Answer from the drawing. Dimensions are ordinates in mm from the lowest x, y and z of the part. Round coordinates to 2 decimals unless told otherwise and drop trailing zeros. Loops run counter-clockwise (first coordinate to the right, second up) from the corner with the lowest first, then second, coordinate; pieces in that order, holes last. Notation, with made-up numbers: (77.25, -5.75) - (109.25, -5.75) arc R22 cw to (109.25, 16.25) - close; hole circle Ø9 at (17, -11.5). An arc over 180 degrees is marked (long way). Write item = value, one per line. Start each with the question number.
1) Section C-C, the plane y = 13 is taken. Determine the outline of the cut face in (x, z) (3 decimals), and give its area (3 significant figures).
2) Section A-A, the plane y = 21 is taken. Determine the outline of the cut face in (x, z), and give its area (3 significant figures).
3) Section D-D, the plane z = 20.5 is taken. Determine the outline of the cut face in (x, y), and give its area (3 significant figures).
4) Section B-B, the plane x = 2.7 is taken. Determine the outline of the cut face in (y, z) (3 decimals), and give its area (3 significant figures).
5) Straight lines are drawn through the part: line 1 along Y through (x, z) = (1.15, 7.5) (3 decimals); line 2 along Z through (x, y) = (1.05, 41.5); line 3 along Y through (x, z) = (0.75, 55). For each, find the intervals that lie inside material, in ascending order.
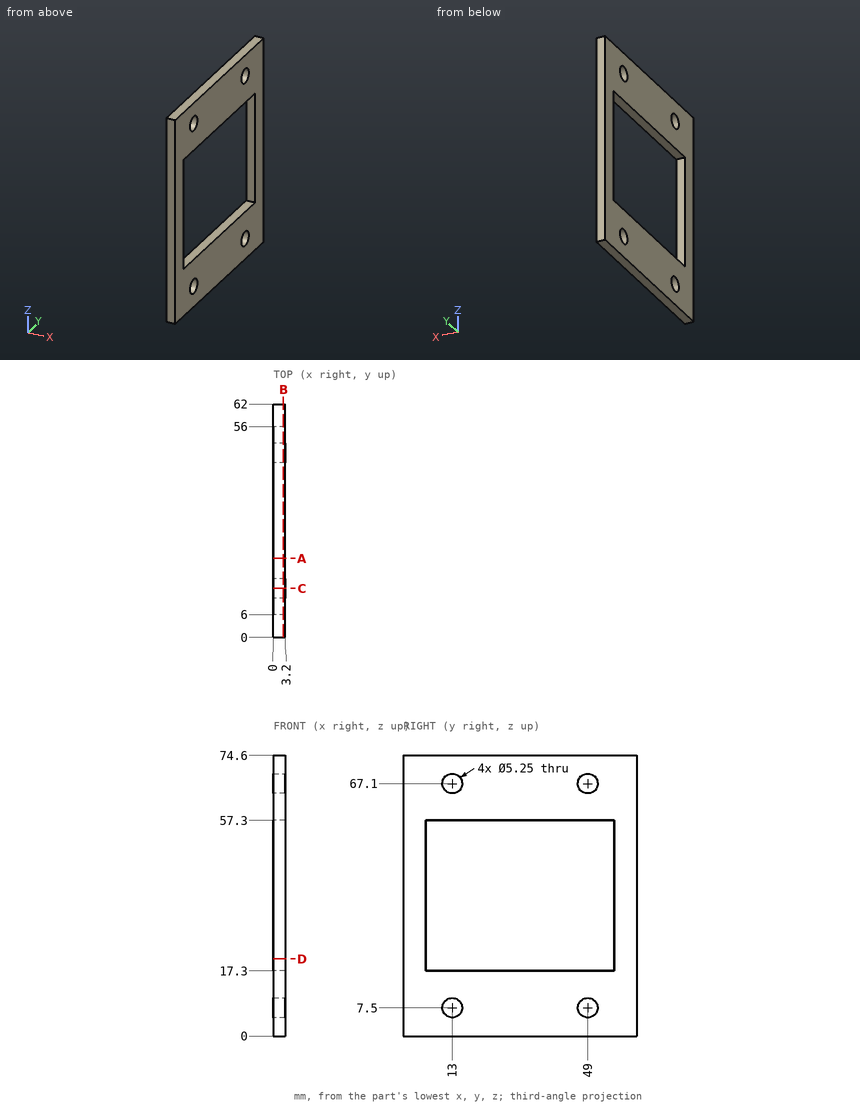
Geometry check:
q1.outline = (0, 0) - (3.2, 0) - (3.2, 4.875) - (0, 4.875) - close; (0, 10.125) - (3.2, 10.125) - (3.2, 17.3) - (0, 17.3) - close; (0, 57.3) - (3.2, 57.3) - (3.2, 64.475) - (0, 64.475) - close; (0, 69.725) - (3.2, 69.725) - (3.2, 74.6) - (0, 74.6) - close
q1.area = 77.1 mm2
q2.outline = (0, 0) - (3.2, 0) - (3.2, 17.3) - (0, 17.3) - close; (0, 57.3) - (3.2, 57.3) - (3.2, 74.6) - (0, 74.6) - close
q2.area = 111 mm2
q3.outline = (0, 0) - (3.2, 0) - (3.2, 6) - (0, 6) - close; (0, 56) - (3.2, 56) - (3.2, 62) - (0, 62) - close
q3.area = 38.4 mm2
q4.outline = (0, 0) - (62, 0) - (62, 74.6) - (0, 74.6) - close; hole (6, 17.3) - (56, 17.3) - (56, 57.3) - (6, 57.3) - close; hole circle Ø5.25 at (13, 7.5); hole circle Ø5.25 at (13, 67.1); hole circle Ø5.25 at (49, 7.5); hole circle Ø5.25 at (49, 67.1)
q4.area = 2,540 mm2
q5.line_1 = 0 to 10.375, 15.625 to 46.375, 51.625 to 62
q5.line_2 = 0 to 17.3, 57.3 to 74.6
q5.line_3 = 0 to 6, 56 to 62
